The listing builds one solid part. Answer for the finished solid, in the listing's coordinates (mm). Give positions to 0.01 mm unless a question says otherwise; leave off trailing zeros. Loops run counter-clockwise (first coordinate to the right, second up) from the corner with the lowest first, then second, coordinate; pieces in that order, holes last. Notation, with made-up numbers: (76.25, -1.5) - (97.25, -1.5) arc R28 ccw to (97.25, 24.5) - close; hole circle Ø3 at (66.25, 45.5). An arc over 180 degrees is marked (long way). Answer as CSV lines item,"result". Start each with the question number.
1) For a pull along Z with two mould halves and no side action, classify faces 1 (the face through (-6, -2, -5)), 2 (the face through (-6, -2, 5)), 3 (the face through (0.748, -8.894, 0.976)), 4 (the face through (-0.748, 8.894, 0.976)) as pulls with the +Z half, pulls with the -Z half, needs draft (parallel to the pull), parting line crosses it, or undercut.
2) A cutting plane is placed at C-C (z = 0.75). Determine the outline of the cut face in (x, y).
3) Find the intervals of material crossed by line 1 along Z through (x, y) = (0, -9.75); line 2 along Y through (x, z) = (0, -2); line 3 along X through (y, z) = (-1.5, 0.5), in increasing order.
4) A cutting plane is placed at D-D (y = 6.5). Determine the outline of the cut face in (x, z).
5) Flat-ended cylindrical pins translate along their axes: pin 1 (2 mm diameter, centred on y = -2.5, z = 0.5, fed in from -X); pin 2 (1.5 mm diameter, centred on x = 0.5, z = 0.5, fed in from +Y). Find the tip coordinate at first contact, or state that the pin passes through.
6) A cutting plane is placed at A-A (x = 0). Determine the outline of the cut face in (y, z).
7) A cutting plane is placed at B-B (y = -3). Determine the outline of the cut face in (x, z), and give its area (3 significant figures).
Autodesk Inventor part; units mm, degrees
ref_plane "Work Plane1" through (12, 0, 0) normal (1, 0, 0) x (0, 1, 0)
ref_plane "XZ Plane" through (0, 0, 0) normal (0, 1, 0) x (-1, 0, 0)
ref_plane "XY Plane" through (0, 0, 0) normal (0, 0, 1) x (1, 0, 0)
sketch "Sketch1" plane through (0, 0, 0) normal (0, 0, 1) x (1, 0, 0)
  circle A0 centre (0, 0) radius 12
  circle A1 centre (0, 0) radius 6
  dimension "d0" = 24
  dimension "d1" = 12
extrude "Extrusion1" add sketch "Sketch1" along normal mid plane 10
thread "Thread1"
ref_plane "Work Plane1" through (12, 0, 0) normal (1, 0, 0) x (0, 1, 0)
sketch "Sketch2" plane through (12, 0, 0) normal (1, 0, 0) x (0, 1, 0)
  point P0 (0, 0)
  point P1 (0, 0)
hole "Hole1" at (12, 0, 0) direction (-1, 0, 0) diameter 2.459 depth 6.5
pattern_circular "Circular Pattern1" count 4 over 360 about axis through (0, 0, 0) along (0, 0, 1) of "Hole1"
properties part number "36" material "Copper"
Ans:
1,face 1,"pulls with the -Z half"
1,face 2,"pulls with the +Z half"
1,face 3,"undercut"
1,face 4,"undercut"
2,outline,"(-11.96, -0.97) arc R12 ccw to (-0.97, -11.96) - (-0.97, -5.92) arc R6 cw to (-5.92, -0.97) - close; (-11.96, 0.97) - (-5.92, 0.97) arc R6 cw to (-0.97, 5.92) - (-0.97, 11.96) arc R12 ccw to start; (0.97, -11.96) arc R12 ccw to (11.96, -0.97) - (5.92, -0.97) arc R6 cw to (0.97, -5.92) - close; (0.97, 5.92) arc R6 cw to (5.92, 0.97) - (11.96, 0.97) arc R12 ccw to (0.97, 11.96) - close"
3,line 1,"-5 to -1.23, 1.23 to 5"
3,line 2,"-12 to -6, 6 to 12"
3,line 3,"-11.91 to -5.81, 5.81 to 11.91"
4,outline,"(-10.09, -5) - (10.09, -5) - (10.09, 5) - (-10.09, 5) - close; hole circle Ø2.46 at (0, 0)"
5,pin 1,"x = -11.91"
5,pin 2,"y = 12"
6,outline,"(-12, -5) - (-6, -5) - (-6, -1.23) - (-12, -1.23) - close; (-12, 1.23) - (-6, 1.23) - (-6, 5) - (-12, 5) - close; (6, -5) - (12, -5) - (12, -1.23) - (6, -1.23) - close; (6, 1.23) - (12, 1.23) - (12, 5) - (6, 5) - close"
7,outline,"(-11.62, -5) - (-5.2, -5) - (-5.2, 5) - (-11.62, 5) - close; (5.2, -5) - (11.62, -5) - (11.62, 5) - (5.2, 5) - close"
7,area,"128 mm2"
